```python
from build123d import *

# Parameters (mm, degrees)
SKETCH1_W           = 76.2
SKETCH1_H           = 101.6
SKETCH1_R           = 3.175
SKETCH1_R_2         = 2.75
BOSS_EXTRUDE1_DEPTH = 9.5
SKETCH_1_R          = 5.25
CUT_EXTRUDE_1_DEPTH = 6.5


with BuildPart() as part:
    # Sketch1 → Boss-Extrude1 (new body)
    with BuildSketch(Plane.XY):
        with Locations((-26.419970967, 29.8958)):
            Rectangle(SKETCH1_W, SKETCH1_H)
        with Locations((-1.019970967, 17.1958)):
            Circle(SKETCH1_R, mode=Mode.SUBTRACT)
        with Locations((-13.719970967, 29.8958)):
            Circle(SKETCH1_R, mode=Mode.SUBTRACT)
        with Locations((-1.019970967, 42.5958)):
            Circle(SKETCH1_R, mode=Mode.SUBTRACT)
        with Locations((-13.719970967, 55.2958)):
            Circle(SKETCH1_R, mode=Mode.SUBTRACT)
        with Locations((-1.019970967, 67.9958)):
            Circle(SKETCH1_R, mode=Mode.SUBTRACT)
        with Locations((-26.419970967, 67.9958)):
            Circle(SKETCH1_R, mode=Mode.SUBTRACT)
        with Locations((-39.119970967, 55.2958)):
            Circle(SKETCH1_R, mode=Mode.SUBTRACT)
        with Locations((-51.819970967, 67.9958)):
            Circle(SKETCH1_R, mode=Mode.SUBTRACT)
        with Locations((-51.819970967, 42.5958)):
            Circle(SKETCH1_R, mode=Mode.SUBTRACT)
        with Locations((-51.819970967, 17.1958)):
            Circle(SKETCH1_R, mode=Mode.SUBTRACT)
        with Locations((-39.119970967, 29.8958)):
            Circle(SKETCH1_R, mode=Mode.SUBTRACT)
        with Locations((-1.019970967, -8.2042)):
            Circle(SKETCH1_R, mode=Mode.SUBTRACT)
        with Locations((-26.419970967, -8.2042)):
            Circle(SKETCH1_R, mode=Mode.SUBTRACT)
        with Locations((-51.819970967, -8.2042)):
            Circle(SKETCH1_R, mode=Mode.SUBTRACT)
        with Locations((-43.169970967, 4.207209087)):
            Circle(SKETCH1_R_2, mode=Mode.SUBTRACT)
        with Locations((-9.669970967, 4.207209087)):
            Circle(SKETCH1_R_2, mode=Mode.SUBTRACT)
        with Locations((-9.669970967, 64.107209087)):
            Circle(SKETCH1_R_2, mode=Mode.SUBTRACT)
        with Locations((-43.169970967, 64.107209087)):
            Circle(SKETCH1_R_2, mode=Mode.SUBTRACT)
    extrude(amount=BOSS_EXTRUDE1_DEPTH)

    # 草图1 → 切除-拉伸1 (cut)
    with BuildSketch(Plane.XY.offset(9.5)):
        with Locations((-51.819970967, -8.2042)):
            Circle(SKETCH_1_R)
        with Locations((-26.419970967, -8.2042)):
            Circle(SKETCH_1_R)
        with Locations((-1.019970967, -8.2042)):
            Circle(SKETCH_1_R)
        with Locations((-1.019970967, 17.1958)):
            Circle(SKETCH_1_R)
        with Locations((-51.819970967, 17.1958)):
            Circle(SKETCH_1_R)
        with Locations((-39.119970967, 29.8958)):
            Circle(SKETCH_1_R)
        with Locations((-13.719970967, 29.8958)):
            Circle(SKETCH_1_R)
        with Locations((-1.019970967, 42.5958)):
            Circle(SKETCH_1_R)
        with Locations((-51.819970967, 42.5958)):
            Circle(SKETCH_1_R)
        with Locations((-39.119970967, 55.2958)):
            Circle(SKETCH_1_R)
        with Locations((-13.719970967, 55.2958)):
            Circle(SKETCH_1_R)
        with Locations((-1.019970967, 67.9958)):
            Circle(SKETCH_1_R)
        with Locations((-26.419970967, 67.9958)):
            Circle(SKETCH_1_R)
        with Locations((-51.819970967, 67.9958)):
            Circle(SKETCH_1_R)
    extrude(amount=-CUT_EXTRUDE_1_DEPTH, mode=Mode.SUBTRACT)


solid = part.part
```
Verification items for the finished model (mm, model axes). A direction names the side the tool comes from. Give positions to 0.01 mm unless a question says otherwise; leave off trailing zeros. Order: outer loops, then holes, each group sorted by start corner. A loop starts at its lowest first (then second) coordinate and runs counter-clockwise, first axis right, second up. Notation, with made-up numbers: (4, 5) -> (10, 5) arc R14 cw to (10, 13) -> close; hole circle Ø2 at (-17.5, 40.5). An arc over 180 degrees is marked (long way). Use a Markdown table: item, result.
1) Mould release check, pull along Y, two halves, no side actions. Record for faces 3 (the flat face through (-64.52, 29, 5)), 4 (the flat face through (-27, -20.904, 5)), 5 (the cylindrical face through (-48.887, -9.42, 1.479)): pulls with the +Y half, pulls with the -Y half, needs draft (parallel to the pull), parting line crosses it, or undercut.
Results:
| item | result |
|---|---|
| face 3 | needs draft |
| face 4 | pulls with the -Y half |
| face 5 | undercut |
2) Section check B-B, the plane z = 1.5. Give the number of separate pieces and of enclosed holes in the cut face, then the cut area to 3 significant figures.
Results:
| item | result |
|---|---|
| separate pieces | 1 |
| enclosed holes | 18 |
| area | 7,200 mm² |
3) Section check C-C, the plane y = 69.5. Record the boundary of the cut face in (x, z).
Results:
| item | result |
|---|---|
| outline | (-64.52, 0) -> (-54.62, 0) -> (-54.62, 3) -> (-56.85, 3) -> (-56.85, 9.5) -> (-64.52, 9.5) -> close; (-49.02, 0) -> (-29.22, 0) -> (-29.22, 3) -> (-31.45, 3) -> (-31.45, 9.5) -> (-46.79, 9.5) -> (-46.79, 3) -> (-49.02, 3) -> close; (-23.62, 0) -> (-3.82, 0) -> (-3.82, 3) -> (-6.05, 3) -> (-6.05, 9.5) -> (-21.39, 9.5) -> (-21.39, 3) -> (-23.62, 3) -> close; (1.78, 0) -> (11.68, 0) -> (11.68, 9.5) -> (4.01, 9.5) -> (4.01, 3) -> (1.78, 3) -> close |
4) Section check A-A, the plane y = 41. Record the boundary of the cut face in (x, z).
Results:
| item | result |
|---|---|
| outline | (-64.52, 0) -> (-54.56, 0) -> (-54.56, 3) -> (-56.82, 3) -> (-56.82, 9.5) -> (-64.52, 9.5) -> close; (-49.08, 0) -> (-3.76, 0) -> (-3.76, 3) -> (-6.02, 3) -> (-6.02, 9.5) -> (-46.82, 9.5) -> (-46.82, 3) -> (-49.08, 3) -> close; (1.72, 0) -> (11.68, 0) -> (11.68, 9.5) -> (3.98, 9.5) -> (3.98, 3) -> (1.72, 3) -> close |
5) Depth check by flat-ended pin: pin 1 Ø8.5 at (x, y) = (-51.82, 17.2) entering from -Z; pin 2 Ø5 at (x, y) = (-50, 44) entering from +Z. Enter the tip coordinate at first touch or a pass-through.
Results:
| item | result |
|---|---|
| pin 1 | z = 0 |
| pin 2 | z = 3 |
6) Tool access check on faces 1 (the cylindrical face through (-48.887, 66.78, 1.479)), 2 (the cylindrical face through (-43.286, 52.101, 6.296)). Record the directions out of +Z, -Z, +X, -X, +Y, -Y that give a thin tool (end or side, any length) a straight path to the whole face; none if there is none.
Results:
| item | result |
|---|---|
| face 1 | +Z, -Z |
| face 2 | +Z |
7) Material ranges on probe 1 along Y at (x, z) = (-26, 8.25); probe 2 along X at (y, z) = (4, 7.75); probe 3 along X at (y, z) = (17, 6.5), recorded low to high.
Results:
| item | result |
|---|---|
| probe 1 | -20.9 to -13.44, -2.97 to 62.76, 73.23 to 80.7 |
| probe 2 | -64.52 to -45.91, -40.43 to -12.41, -6.93 to 11.68 |
| probe 3 | -64.52 to -57.07, -46.57 to -6.27, 4.23 to 11.68 |
